```python
from build123d import *

# Parameters (mm, degrees)
SKETCH1_R           = 2.4892
BOSS_EXTRUDE1_DEPTH = 49.2125
SKETCH2_OUTSIDE_W   = 36.728
SKETCH2_OUTSIDE_H   = 34.764
SKETCH2_OUTSIDE_R   = 6.35
CUT_EXTRUDE1_DEPTH  = 7.9375


with BuildPart() as part:
    # Sketch1 → Boss-Extrude1 (new, symmetric)
    with BuildSketch(Plane.XY):
        Polygon((3.666174209, 6.35), (-3.666174209, 6.35), (-7.332348419, 0), (-3.666174209, -6.35), (3.666174209, -6.35), (7.332348419, 0), align=None)
        Circle(SKETCH1_R, mode=Mode.SUBTRACT)
    extrude(amount=BOSS_EXTRUDE1_DEPTH, both=True)

    # Sketch2 outside → Cut-Extrude1 (cut)
    with BuildSketch(Plane.XY.offset(49.2125)):
        Rectangle(SKETCH2_OUTSIDE_W, SKETCH2_OUTSIDE_H)
        Circle(SKETCH2_OUTSIDE_R, mode=Mode.SUBTRACT)
    cut_extrude1 = extrude(amount=-CUT_EXTRUDE1_DEPTH, mode=Mode.SUBTRACT)

    # Mirror1: Cut-Extrude1 across plane
    add(cut_extrude1.mirror(Plane.XY), mode=Mode.SUBTRACT)


solid = part.part
```
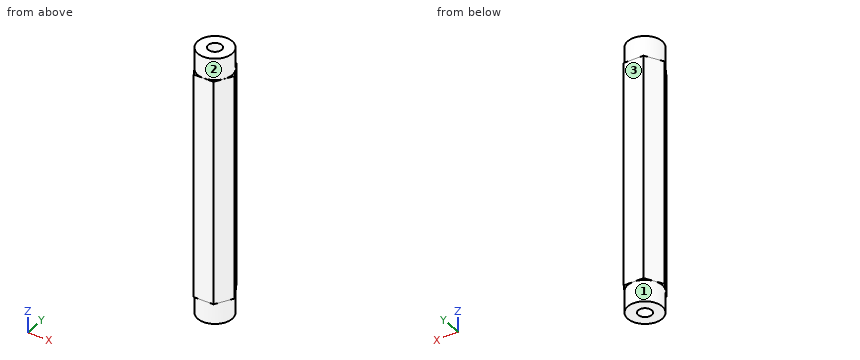
For this review, take the finished solid that the model builds, in its own axes (mm). Face numbers are marked on the shaded views. A direction names the side the tool comes from. Coordinates: 2 decimals unless noted, no trailing zeros. Order: outer loops, then holes, each group sorted by start corner. A loop starts at its lowest first (then second) coordinate and runs counter-clockwise, first axis right, second up. Notation, with made-up numbers: (-6, 81) - (11, 81) arc R12 ccw to (11, 93) - close; hole circle Ø11 at (76, 8). An arc over 180 degrees is marked (long way). Answer as a JSON object with one key per item and string values. Group by question number.
1. For probe 1 along Z at (x, y) = (6, 2.25) (3 decimals); probe 2 along X at (y, z) = (2, -26.5); probe 3 along X at (y, z) = (0.75, -27.5), list the stretches that pass through material, from the lowest coordinate up.
2. Clearance check with a flat-ended pin moving along its axis: P1, Ø1, axis at y = 3.5, z = -16.5, coming from the +X side. State where the tip first meets the part, or that it passes through.
3. We need section A-A on z = -33. State the section outline as (x, y) points, then the cut area to 3 significant figures.
4. For the marked faces 1, 2 and 3, list the 3-axis set-ups (+Z, -Z, +X, -X, +Y, -Y) from which the entire face can be reached by the end or side of a thin tool; tool diameter is ignored.
Final values:
{
 "1": {"probe 1": "-41.275 to 41.275", "probe 2": "-6.18 to -1.48, 1.48 to 6.18", "probe 3": "-6.9 to -2.37, 2.37 to 6.9"},
 "2": {"P1": "x = 5.6"},
 "3": {"outline": "(-7.33, 0) - (-3.67, -6.35) - (3.67, -6.35) - (7.33, 0) - (3.67, 6.35) - (-3.67, 6.35) - close; hole circle Ø4.98 at (0, 0)", "area": "120 mm²"},
 "4": {"face 1": "-Z", "face 2": "+Z", "face 3": "+Z, -Z, +X, -X, +Y"}
}
